Job drawing, mm, ordinate dimensions from the low corner. One solid piece. Give positions to 0.01 mm unless a question says otherwise; leave off trailing zeros. Loops run counter-clockwise (first coordinate to the right, second up) from the corner with the lowest first, then second, coordinate; pieces in that order, holes last.
Item 1: Probe probe 1 along X at (y, z) = (25.5, 27); probe 2 along Y at (x, z) = (75, 22); probe 3 along X at (y, z) = (31, 40). List the from-to ranges inside material, lowest first.
Item 2: Mould opens along Z. For the marked faces 1, 2, 3 and 4 say: released by +Z, released by -Z, zero draft, split by the parting line, or undercut.
Item 3: Saw through at D-D on y = 52. Give the cut face in (x, z), plus the area to 3 significant figures.
Item 4: Saw through at C-C on y = 33. Give the cut face in (x, z), plus the area to 3 significant figures.
Item 5: Saw through at A-A on x = 15. Give the cut face in (y, z).
Item 6: Drop flat-ended pins along their axis: P1, Ø4, axis at y = 27.5, z = 43.5, coming from the -X side; P2, Ø10, axis at x = 63.5, z = 51, coming from the +Y side; P3, Ø6, axis at x = 24, y = 22.5, coming from the -Z side. Give the stop position or say it passes through.
Item 7: Saw through at B-B on z = 41.5. Give the cut face in (x, y), plus the area to 3 significant figures.
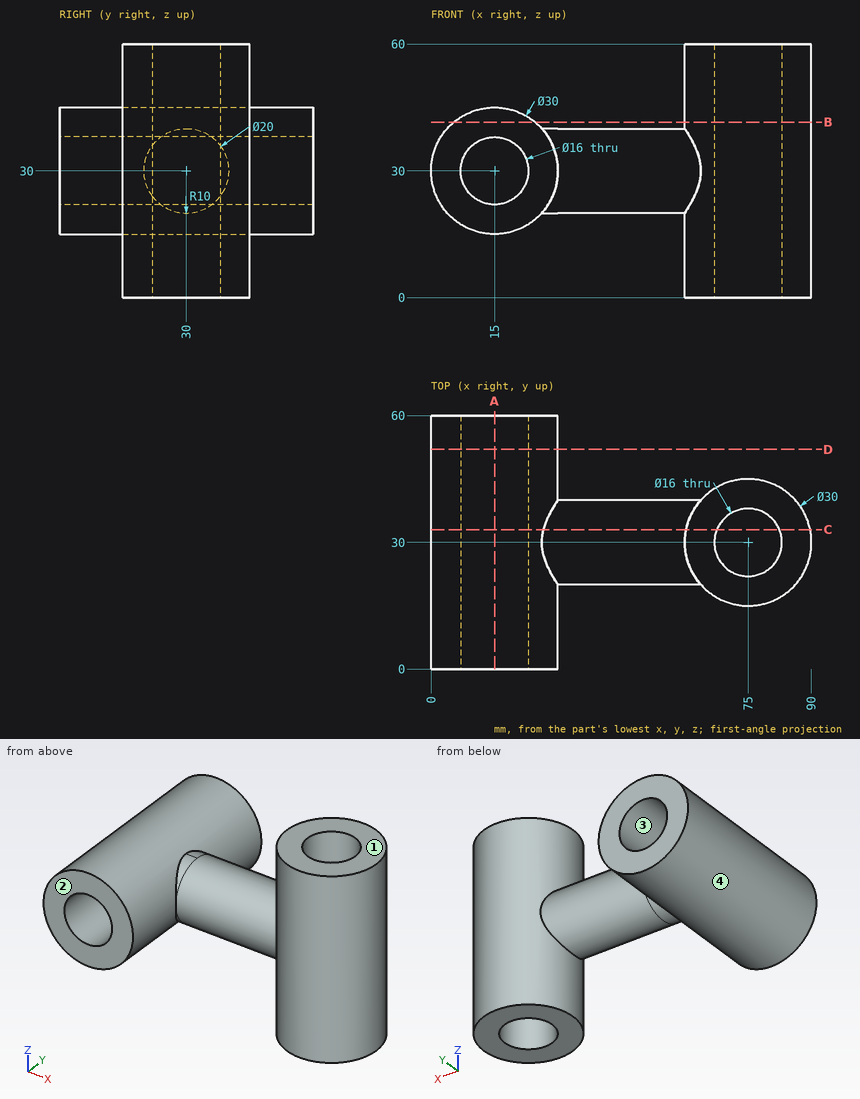
Results below:
1. probe 1: x = 0.3 to 7.58, 22.42 to 68.39, 81.61 to 89.31
1. probe 2: y = 15 to 22, 38 to 45
1. probe 3: x = 3.82 to 26.18, 60.03 to 67.06, 82.94 to 89.97
2. face 1: released by +Z
2. face 2: zero draft
2. face 3: undercut
2. face 4: split by the parting line
3. outline: circle Ø30 at (15, 30); hole circle Ø16 at (15, 30)
3. area: 506 mm2
4. outline: (26.58, 20.46) - (60.3, 20.46) - (60.3, 0) - (67.58, 0) - (67.58, 60) - (60.3, 60) - (60.3, 39.54) - (26.58, 39.54) arc R15 ccw (long way) to start; (82.42, 0) - (89.7, 0) - (89.7, 60) - (82.42, 60) - close; hole circle Ø16 at (15, 30)
4. area: 1,980 mm2
5. outline: (0, 15) - (60, 15) - (60, 22) - (0, 22) - close; (0, 38) - (60, 38) - (60, 45) - (0, 45) - close
6. P1: stops at x = 5.37
6. P2: stops at y = 43.52
6. P3: stops at z = 16.25
7. outline: (5.37, 0) - (24.63, 0) - (24.63, 60) - (5.37, 60) - close; circle Ø30 at (75, 30); hole circle Ø16 at (75, 30)
7. area: 1,660 mm2
